from build123d import *

# Parameters (mm, degrees)
SKETCH1_W           = 70
SKETCH1_H           = 15
BOSS_EXTRUDE1_DEPTH = 3
SKETCH2_W           = 3
SKETCH2_H           = 15
BOSS_EXTRUDE2_DEPTH = 75
CUT_EXTRUDE1_DEPTH  = 75
SKETCH4_W           = 70
SKETCH4_H           = 18.892094127
BOSS_EXTRUDE3_DEPTH = 3


with BuildPart() as part:
    # Sketch1 → Boss-Extrude1 (new body)
    with BuildSketch(Plane.XY):
        with Locations((83.09202796, -33.31343354)):
            Rectangle(SKETCH1_W, SKETCH1_H)
    extrude(amount=BOSS_EXTRUDE1_DEPTH)

    # Sketch2 → Boss-Extrude2 (add)
    with BuildSketch(Plane.XY.offset(3)):
        with Locations((49.59202796, -33.31343354)):
            Rectangle(SKETCH2_W, SKETCH2_H)
        with Locations((116.59202796, -33.31343354)):
            Rectangle(SKETCH2_W, SKETCH2_H)
    extrude(amount=BOSS_EXTRUDE2_DEPTH)

    # Sketch3 → Cut-Extrude1 (cut)
    with BuildSketch(Plane.ZY.offset(-48.09202796)):
        Polygon((0, -40.81343354), (78, -40.81343354), (68, -35.81343354), (0, -35.81343354), align=None)
    extrude(amount=-CUT_EXTRUDE1_DEPTH, mode=Mode.SUBTRACT)

    # Sketch4 → Boss-Extrude3 (add)
    with BuildSketch(Plane(origin=(0, -25.81343354, 0), x_dir=(1, 0, 0), z_dir=(0, 1, 0))):
        with Locations((83.09202796, -36.511528279)):
            Rectangle(SKETCH4_W, SKETCH4_H)
    extrude(amount=BOSS_EXTRUDE3_DEPTH)


solid = part.part
Geometry check sheet. Reference: the model listing, model coordinates, mm. A direction names the side the tool comes from. Give positions to 0.01 mm unless a question says otherwise; leave off trailing zeros. Write each loop counter-clockwise with the first axis right and the second up, starting at its lowest first coordinate (ties: lowest second). Pieces come first, ordered by that corner, then holes.
1) Cross-section at D-D (z = 35.5). Record the boundary of the cut face in (x, y).
Values follow:
outline: (48.09, -35.81) - (51.09, -35.81) - (51.09, -25.81) - (115.09, -25.81) - (115.09, -35.81) - (118.09, -35.81) - (118.09, -22.81) - (48.09, -22.81) - close
2) Cross-section at B-B (x = 96). Record the boundary of the cut face in (y, z).
Values follow:
outline: (-35.81, 0) - (-25.81, 0) - (-25.81, 3) - (-35.81, 3) - close; (-25.81, 27.07) - (-22.81, 27.07) - (-22.81, 45.96) - (-25.81, 45.96) - close
3) Thickness scan on line 1 (X direction, y = -34.25, z = 34.5); line 2 (Z direction, x = 72.5, y = -29.5); line 3 (Y direction, x = 68, z = 43.5). Record the ranges inside material, lowest first.
Values follow:
line 1: x = 48.09 to 51.09, 115.09 to 118.09
line 2: z = 0 to 3
line 3: y = -25.81 to -22.81
4) Cross-section at C-C (y = -34.25). Record the boundary of the cut face in (x, z).
Values follow:
outline: (48.09, 0) - (118.09, 0) - (118.09, 78) - (115.09, 78) - (115.09, 3) - (51.09, 3) - (51.09, 78) - (48.09, 78) - close
5) Release check for a two-part mould opening along X. For faces 1 (the face through (118.092, -30, 40)), 2 (the face through (115.092, -32, 40)), 3 (the face through (83, -35.813, 1)), 4 (the face through (51.092, -32, 40)) record: released by +X, released by -X, zero draft, split by the parting line, or undercut.
Values follow:
face 1: released by +X
face 2: undercut
face 3: zero draft
face 4: undercut
6) Cross-section at A-A (z = 60.5). Record the boundary of the cut face in (x, y), plus the area to 3 significant figures.
Values follow:
outline: (48.09, -35.81) - (51.09, -35.81) - (51.09, -25.81) - (48.09, -25.81) - close; (115.09, -35.81) - (118.09, -35.81) - (118.09, -25.81) - (115.09, -25.81) - close
area: 60.0 mm2
7) Go/stop test with flat-tipped pins: pin 1 Ø10 at (x, y) = (79, -38) entering from +Z; pin 2 Ø9.5 at (x, z) = (98, 37) entering from -Y; pin 3 Ø1.5 at (x, z) = (49.5, 55.5) entering from +Y; pin 4 Ø2 at (y, z) = (-36.5, 31.5) entering from +X. Record where each tip stops, or that it passes through.
Values follow:
pin 1: stops at z = 3
pin 2: stops at y = -25.81
pin 3: stops at y = -25.81
pin 4: stops at x = 118.09
8) Set-up check for faces 5 (the face through (83, -25.813, 36)), 6 (the face through (83, -25.813, 2)), 7 (the face through (83, -31, 3)): record each of +Z, -Z, +X, -X, +Y, -Y from which the full face is reachable in a straight line by a thin tool's end or side.
Values follow:
face 5: +Z, -Y
face 6: -Z, +X, -X, +Y
face 7: +Z, +Y, -Y
